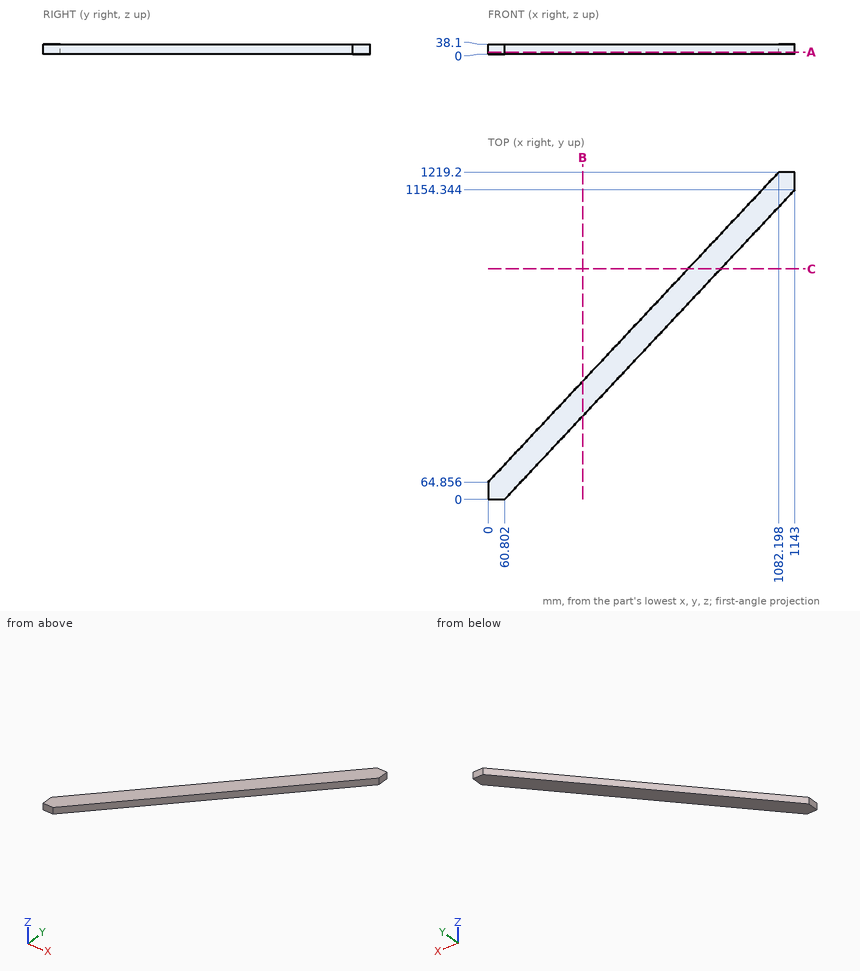
Part print with two shaded views. Sizes in mm from the minimum x, y, z corner. Round coordinates to 2 decimals unless told otherwise and drop trailing zeros. Order: outer loops, then holes, each group sorted by start corner. A loop starts at its lowest first (then second) coordinate and runs counter-clockwise, first axis right, second up. Notation, with made-up numbers: (86.25, 35) - (116.25, 35) arc R5 ccw to (116.25, 44) - close; hole circle Ø11 at (-27.75, -9). An arc over 180 degrees is marked (long way). Return JSON: item names as keys, results as strings.
(1) Pin check, flat tips, straight feed: pin 1 Ø2 at (y, z) = (694, 21.5) entering from -X (1 decimal); pin 2 Ø8 at (y, z) = (1008, 33.5) entering from -X; pin 3 Ø12 at (y, z) = (1092, 25.5) entering from +X. Stop position of each tip, or through.
Answer key:
{"pin 1": "stops at x = 588.9", "pin 2": "stops at x = 880.45", "pin 3": "stops at x = 1090.18"}
(2) Cut at C-C (y = 859). Give the cut face in (x, z) (1 decimal), then the cut area to 3 significant figures.
Answer key:
{"outline": "(744.5, 0) - (866.1, 0) - (866.1, 38.1) - (744.5, 38.1) - close", "area": "4,630 mm^2"}
(3) Cut at A-A (z = 7.5). Give the cut face in (x, y), then the cut area to 3 significant figures.
Answer key:
{"outline": "(0, 0) - (60.8, 0) - (1143, 1154.34) - (1143, 1219.2) - (1082.2, 1219.2) - (0, 64.86) - close", "area": "144,000 mm^2"}
(4) Cut at B-B (x = 352). Give the cut face in (y, z), then the cut area to 3 significant figures.
Answer key:
{"outline": "(310.61, 0) - (440.32, 0) - (440.32, 38.1) - (310.61, 38.1) - close", "area": "4,940 mm^2"}
(5) Wall check: probe 1 along Y at (x, z) = (326, 36) (1 decimal); probe 2 along Y at (x, z) = (897, 22.5) (1 decimal); probe 3 along X at (y, z) = (472, 26). Give the ranges that are in metal, low to high. Write a range as from..to.
Answer key:
{"probe 1": "y = 282.9..412.6", "probe 2": "y = 891.9..1021.7", "probe 3": "x = 381.7..503.3"}
